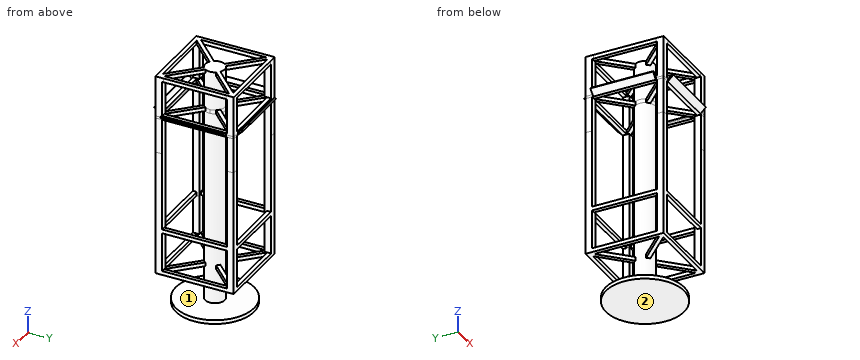
```python
from build123d import *

# Parameters (mm, degrees)
F0_R           = 304.8
F1_DEPTH       = 30.48
F2_R           = 76.2
F3_DEPTH       = 274.32
F4_W           = 609.6
F4_H           = 609.6
F5_DEPTH       = 30.48
F6_R           = 76.2
F6_W           = 52.0326146906
F6_H           = 52.0326146906
F7_DEPTH       = 304.8
F7_DEPTH_BACK  = 30.48
F8_W           = 609.6
F8_H           = 609.6
F8_W_2         = 548.64
F8_H_2         = 548.64
F9_DEPTH       = 30.48
F10_W          = 52.4256
F10_H          = 52.4256
F10_R          = 76.2
F11_DEPTH      = 914.4
F13_DEPTH      = 30.48
F14_W          = 52.4256
F14_H          = 52.4256
F14_R          = 76.2
F15_DEPTH      = 304.8
F15_DEPTH_BACK = 30.48
F16_W          = 609.6
F16_H          = 609.6
F16_W_2        = 548.64
F16_H_2        = 548.64
F17_DEPTH      = 30.48
F20_DEPTH      = 609.6
F22_DEPTH      = 609.6
F23_DEPTH      = 30.48
F24_W          = 60.96
F24_H          = 72.17660923
F24_H_2        = 60.96
F24_H_3        = 74.9131180763
F24_W_2        = 86.0498287201
F24_W_3        = 73.7356283188
F24_H_4        = 73.4948553562
F24_H_5        = 80.3360976696
F24_W_4        = 73.3040608883
F25_DEPTH      = 609.6


# Not quite as in the source:
# - a feature names something its author has since deleted; it is built from what else it names


with BuildPart() as f1:
    # F0 (on Top) → F1 (new body)
    with BuildSketch(Plane.XY):
        Circle(F0_R)
    extrude(amount=F1_DEPTH)

    # F2 (on face) → F3 (join)
    with BuildSketch(Plane.XY.offset(30.48)):
        Circle(F2_R)
    extrude(amount=F3_DEPTH)

    # F4 (on face) → F5 (join)
    with BuildSketch(Plane.XY.offset(304.8)):
        Rectangle(F4_W, F4_H)
        Polygon((-21.5526146906, 0), (-274.32, -252.7673853094), (-274.32, 252.7673853094), align=None, mode=Mode.SUBTRACT)
        Polygon((0, -21.5526146906), (252.7673853094, -274.32), (-252.7673853094, -274.32), align=None, mode=Mode.SUBTRACT)
        Polygon((-252.7673853094, 274.32), (252.7673853094, 274.32), (0, 21.5526146906), align=None, mode=Mode.SUBTRACT)
        Polygon((274.32, 252.7673853094), (274.32, -252.7673853094), (21.5526146906, 0), align=None, mode=Mode.SUBTRACT)
    extrude(amount=F5_DEPTH)

    # F6 (on face) → F7 (join, two sides)
    with BuildSketch(Plane.XY.offset(335.28)) as f7_sk:
        Circle(F6_R)
        with Locations((-278.7836926547, 278.7836926547)):
            Rectangle(F6_W, F6_H)
        with Locations((278.7836926547, 278.7836926547)):
            Rectangle(F6_W, F6_H)
        with Locations((278.7836926547, -278.7836926547)):
            Rectangle(F6_W, F6_H)
        with Locations((-278.7836926547, -278.7836926547)):
            Rectangle(F6_W, F6_H)
    extrude(amount=F7_DEPTH)
    extrude(f7_sk.sketch, amount=-F7_DEPTH_BACK)

    # F8 (on face) → F9 (join)
    with BuildSketch(Plane.XY.offset(640.08)):
        Rectangle(F8_W, F8_H)
        Rectangle(F8_W_2, F8_H_2, mode=Mode.SUBTRACT)
    extrude(amount=F9_DEPTH)

    # F10 (on face) → F11 (join)
    with BuildSketch(Plane.XY.offset(640.08)):
        with Locations((-278.5872, 278.5872)):
            Rectangle(F10_W, F10_H)
        with Locations((-278.5872, -278.5872)):
            Rectangle(F10_W, F10_H)
        with Locations((278.5872, 278.5872)):
            Rectangle(F10_W, F10_H)
        with Locations((278.5872, -278.5872)):
            Rectangle(F10_W, F10_H)
        Circle(F10_R)
    extrude(amount=F11_DEPTH)

    # F12 (on face) → F13 (join)
    with BuildSketch(Plane.XY.offset(1554.48)):
        Polygon((252.3744, -304.8), (304.8, -304.8), (304.8, -252.3744), (304.8, 252.3744), (304.8, 304.8), (252.3744, 304.8), (-252.3744, 304.8), (-304.8, 304.8), (-304.8, 252.3744), (-304.8, -252.3744), (-304.8, -304.8), (-252.3744, -304.8), align=None)
        Polygon((252.3744, -274.32), (-252.3744, -274.32), (0, -21.9456), align=None, mode=Mode.SUBTRACT)
        Polygon((-274.32, -252.3744), (-274.32, 252.3744), (-21.9456, 0), align=None, mode=Mode.SUBTRACT)
        Polygon((21.9456, 0), (274.32, 252.3744), (274.32, -252.3744), align=None, mode=Mode.SUBTRACT)
        Polygon((0, 21.9456), (-252.3744, 274.32), (252.3744, 274.32), align=None, mode=Mode.SUBTRACT)
    extrude(amount=F13_DEPTH)

    # F14 (on face) → F15 (join, two sides)
    with BuildSketch(Plane.XY.offset(1584.96)) as f15_sk:
        with Locations((-278.5872, 278.5872)):
            Rectangle(F14_W, F14_H)
        with Locations((278.5872, 278.5872)):
            Rectangle(F14_W, F14_H)
        with Locations((278.5872, -278.5872)):
            Rectangle(F14_W, F14_H)
        with Locations((-278.5872, -278.5872)):
            Rectangle(F14_W, F14_H)
        Circle(F14_R)
    extrude(amount=F15_DEPTH)
    extrude(f15_sk.sketch, amount=-F15_DEPTH_BACK)

    # F16 (on face) → F17 (join)
    with BuildSketch(Plane.XY.offset(1889.76)):
        Rectangle(F16_W, F16_H)
        Rectangle(F16_W_2, F16_H_2, mode=Mode.SUBTRACT)
    extrude(amount=-F17_DEPTH)

    # F19 (on face) → F20 (join)
    with BuildSketch(Plane.XZ.offset(304.8)):
        Polygon((-347.9052293811, 1597.5852293811), (-304.8, 1554.48), (-274.32, 1554.48), (-274.32, 1571.7220917525), (-304.8, 1571.7220917525), (-339.2841835049, 1606.2062752574), align=None)
        Polygon((274.32, 1554.48), (304.8, 1554.48), (347.9052293811, 1597.5852293811), (339.2841835049, 1606.2062752574), (304.8, 1571.7220917525), (274.32, 1571.7220917525), align=None)
    extrude(amount=-F20_DEPTH)

    # F21 (on face) → F22 (join)
    with BuildSketch(Plane.YZ.offset(304.8)):
        Polygon((274.32, 1571.7220917525), (274.32, 1554.48), (304.8, 1554.48), (347.9052293811, 1597.5852293811), (339.2841835049, 1606.2062752574), (304.8, 1571.7220917525), align=None)
        Polygon((-304.8, 1554.48), (-274.32, 1554.48), (-274.32, 1571.7220917525), (-304.8, 1571.7220917525), (-339.2841835049, 1606.2062752574), (-347.9052293811, 1597.5852293811), align=None)
    extrude(amount=-F22_DEPTH)

    # F18 (on face) → F23 (join)
    with BuildSketch(Plane.XY.offset(1889.76)):
        Polygon((0, 21.9456), (-252.3744, 274.32), (-274.32, 274.32), (-274.32, 252.3744), (-21.9456, 0), (-274.32, -252.3744), (-274.32, -274.32), (-252.3744, -274.32), (0, -21.9456), (252.3744, -274.32), (274.32, -274.32), (274.32, -252.3744), (21.9456, 0), (274.32, 252.3744), (274.32, 274.32), (252.3744, 274.32), align=None)
    extrude(amount=-F23_DEPTH)

    # F24 (on face) → F25 (cut)
    with BuildSketch(Plane.XY.offset(1889.76)):
        with Locations((-274.32, 340.888304615)):
            Rectangle(F24_W, F24_H)
        with Locations((-335.28, 274.32)):
            Rectangle(F24_W, F24_H_2)
        with Locations((274.32, 342.2565590382)):
            Rectangle(F24_W, F24_H_3)
        with Locations((347.82491436, 274.32)):
            Rectangle(F24_W_2, F24_H_2)
        with Locations((341.6678141594, -274.32)):
            Rectangle(F24_W_3, F24_H_2)
        with Locations((274.32, -341.5474276781)):
            Rectangle(F24_W, F24_H_4)
        with Locations((-274.32, -344.9680488348)):
            Rectangle(F24_W, F24_H_5)
        with Locations((-341.4520304441, -274.32)):
            Rectangle(F24_W_4, F24_H_2)
    extrude(amount=-F25_DEPTH, mode=Mode.SUBTRACT)


solid = f1.part
```
The listing builds one solid part. Answer for the finished solid, in the listing's coordinates (mm). Face numbers are marked on the shaded views. Round coordinates to 2 decimals unless told otherwise and drop trailing zeros. Write each loop counter-clockwise with the first axis right and the second up, starting at its lowest first coordinate (ties: lowest second). Pieces come first, ordered by that corner, then holes. Notation, with made-up numbers: (-19, -13.75) -> (-4, -13.75) arc R18 ccw to (-4, 17.25) -> close; hole circle Ø11 at (59, 64). An arc over 180 degrees is marked (long way). Answer as a JSON object with one key per item and string values. Group by question number.
Q1. Determine the mould class of the marked faces 1 and 2 for opening direction Z: pulls with the +Z half, pulls with the -Z half, needs draft (parallel to the pull), parting line crosses it, or undercut.
Q2. Each of these flat-tipped pins is pushed along its axis until it touches: pin 1 Ø10 at (x, z) = (-263.5, 1006.5) entering from +Y; pin 2 Ø4 at (y, z) = (-145, 317.5) entering from -X; pin 3 Ø10.5 at (y, z) = (45, 1579.5) entering from +X. Where does it stop, or does it pass through?
Q3. Straight lines are drawn through the part: line 1 along Z through (x, y) = (300, 216.5); line 2 along Z through (x, y) = (-80.5, -89); line 3 along X through (y, z) = (262, 1213). For each, find the intervals that lie inside material, in ascending order.
Q4. Section B-B (z = 964) is taken. Write down the section's boundary in (x, y).
Q5. Section C-C (x = 0) is taken. Count the separate pieces of the cut face and the enclosed holes in it, plus the area to 3 significant figures.
Q6. Section A-A (z = 602.5) is taken. Write down the section's boundary in (x, y), plus the area to 3 significant figures.
Check values:
{
 "1": {"face 1": "undercut", "face 2": "pulls with the -Z half"},
 "2": {"pin 1": "y = 304.8", "pin 2": "x = -304.8", "pin 3": "x = 335.07"},
 "3": {"line 1": "304.8 to 335.28, 640.08 to 670.56, 1554.48 to 1584.96, 1859.28 to 1889.76", "line 2": "0 to 30.48, 304.8 to 335.28, 1554.48 to 1584.96, 1859.28 to 1889.76", "line 3": "-304.8 to -252.37, 252.37 to 304.8"},
 "4": {"outline": "(-304.8, -304.8) -> (-252.37, -304.8) -> (-252.37, -252.37) -> (-304.8, -252.37) -> close; (-304.8, 252.37) -> (-252.37, 252.37) -> (-252.37, 304.8) -> (-304.8, 304.8) -> close; circle Ø152.4 at (0, 0); (252.37, -304.8) -> (304.8, -304.8) -> (304.8, -252.37) -> (252.37, -252.37) -> close; (252.37, 252.37) -> (304.8, 252.37) -> (304.8, 304.8) -> (252.37, 304.8) -> close"},
 "5": {"separate pieces": "9", "enclosed holes": "0", "area": "311,000 mm^2"},
 "6": {"outline": "(-304.8, -304.8) -> (-252.77, -304.8) -> (-252.77, -252.77) -> (-304.8, -252.77) -> close; (-304.8, 252.77) -> (-252.77, 252.77) -> (-252.77, 304.8) -> (-304.8, 304.8) -> close; circle Ø152.4 at (0, 0); (252.77, -304.8) -> (304.8, -304.8) -> (304.8, -252.77) -> (252.77, -252.77) -> close; (252.77, 252.77) -> (304.8, 252.77) -> (304.8, 304.8) -> (252.77, 304.8) -> close", "area": "29,100 mm^2"}
}
